```python
from build123d import *

# Parameters (mm, degrees)
CROQUIS1_R              = 1.500000078
CROQUIS1_R_2            = 0.899999978
CROQUIS1_R_3            = 0.899999104
CROQUIS1_R_4            = 1.499997939
CROQUIS1_R_5            = 1.500000378
SALIENTE_EXTRUIR1_DEPTH = 4
CROQUIS2_R              = 1.500000078
CROQUIS2_R_2            = 0.899999978
CROQUIS2_R_3            = 0.899999104
SALIENTE_EXTRUIR2_DEPTH = 4
CROQUIS3_W              = 35.500002289
CROQUIS3_H              = 4.004000187
SALIENTE_EXTRUIR3_DEPTH = 4
CROQUIS4_W              = 38.100002289
CROQUIS4_H              = 4.004000187
SALIENTE_EXTRUIR4_DEPTH = 8
CROQUIS5_R              = 3
CORTAR_EXTRUIR1_DEPTH   = 8


with BuildPart() as part:
    # Croquis1 → Saliente-Extruir1 (new body)
    with BuildSketch(Plane(origin=(0, 0, 0), x_dir=(1, 0, 0), z_dir=(0, 1, 0))):
        with BuildLine():
            Line((-19.24526482, -19.128405422), (20.25473518, -19.128405422))
            ThreePointArc((20.25473518, -19.128405422), (23.250093999, -17.982284574), (24.715306469, -15.12940535))
            Line((24.715306469, -15.12940535), (24.75473518, 3.871594578))
            ThreePointArc((24.75473518, 3.871594578), (24.41495197, 5.657410091), (23.436719128, 7.189614445))
            Line((23.436719128, 7.189614445), (9.132638286, 18.858517697))
            ThreePointArc((9.132638286, 18.858517697), (7.79788024, 19.61076911), (6.288102337, 19.871598393))
            Line((6.288102337, 19.871598393), (-5.278630069, 19.871598393))
            ThreePointArc((-5.278630069, 19.871598393), (-7.047350485, 19.518737385), (-8.545265011, 18.514180332))
            Line((-8.545265011, 18.514180332), (-22.427247654, 7.189612922))
            ThreePointArc((-22.427247654, 7.189612922), (-23.487263037, 5.764725879), (-23.74526482, 4.007634312))
            Line((-23.74526482, 4.007634312), (-23.68986282, -15.332360357))
            ThreePointArc((-23.68986282, -15.332360357), (-22.167781266, -18.050232235), (-19.24526482, -19.128405422))
        make_face()
        with Locations((-10.945264306, -0.628405976)):
            Circle(CROQUIS1_R, mode=Mode.SUBTRACT)
        with Locations((-6.745264379, -0.628405738)):
            Circle(CROQUIS1_R_2, mode=Mode.SUBTRACT)
        with Locations((21.754736572, -0.628405422)):
            Circle(CROQUIS1_R_3, mode=Mode.SUBTRACT)
        with Locations((6.25473312, 16.341597706)):
            Circle(CROQUIS1_R_4, mode=Mode.SUBTRACT)
        with Locations((-4.945262866, 16.341595261)):
            Circle(CROQUIS1_R_5, mode=Mode.SUBTRACT)
        Polygon((-3.845263294, 5.821595341), (-3.74526482, -15.124405235), (5.25473518, -15.124405235), (5.25473518, -7.078405231), (18.854737469, -7.078405231), (18.854737469, 5.821595341), align=None, mode=Mode.SUBTRACT)
    extrude(amount=SALIENTE_EXTRUIR1_DEPTH)

    # Croquis2 → Saliente-Extruir2 (add)
    with BuildSketch(Plane(origin=(0, 4, 0), x_dir=(1, 0, 0), z_dir=(0, 1, 0))):
        with BuildLine():
            Line((-3.74526482, -15.124405235), (-3.835972877, 3.875594765))
            Line((-3.835972877, 3.875594765), (-14.735972877, 3.875594765))
            Line((-14.735972877, 3.875594765), (-14.735972877, -15.124405235))
            Line((-14.735972877, -15.124405235), (-19.24526482, -15.124405235))
            Line((-19.24526482, -15.124405235), (-19.24526482, -19.128405422))
            Line((-19.24526482, -19.128405422), (20.25473518, -19.128405422))
            ThreePointArc((20.25473518, -19.128405422), (23.250093999, -17.982284574), (24.715306469, -15.12940535))
            Line((24.715306469, -15.12940535), (24.75473518, 3.871594578))
            Line((24.75473518, 3.871594578), (18.854737469, 3.871594578))
            Line((18.854737469, 3.871594578), (18.854737469, -7.078405231))
            Line((18.854737469, -7.078405231), (18.854737469, -15.124405235))
            Line((18.854737469, -15.124405235), (5.25473518, -15.124405235))
            Line((5.25473518, -15.124405235), (-3.74526482, -15.124405235))
        make_face()
        with Locations((-10.945264306, -0.628405976)):
            Circle(CROQUIS2_R, mode=Mode.SUBTRACT)
        with Locations((-6.745264379, -0.628405738)):
            Circle(CROQUIS2_R_2, mode=Mode.SUBTRACT)
        with Locations((21.754736572, -0.628405422)):
            Circle(CROQUIS2_R_3, mode=Mode.SUBTRACT)
    extrude(amount=SALIENTE_EXTRUIR2_DEPTH)

    # Croquis3 → Saliente-Extruir3 (add)
    with BuildSketch(Plane(origin=(0, 8, 0), x_dir=(1, 0, 0), z_dir=(0, 1, 0))):
        with Locations((-1.495263676, -17.126405328)):
            Rectangle(CROQUIS3_W, CROQUIS3_H)
    extrude(amount=SALIENTE_EXTRUIR3_DEPTH)

    # Croquis4 → Saliente-Extruir4 (add)
    with BuildSketch(Plane.XZ):
        with Locations((-0.195263676, 17.126405328)):
            Rectangle(CROQUIS4_W, CROQUIS4_H)
    extrude(amount=SALIENTE_EXTRUIR4_DEPTH)

    # Croquis5 → Cortar-Extruir1 (cut)
    with BuildSketch(Plane.XY.offset(19.128405422)):
        with Locations((-0.195262531, 2)):
            Circle(CROQUIS5_R)
        Polygon((16.254737469, 8), (12.254737469, 12), (16.254737469, 12), align=None)
        Polygon((-19.24526482, 4), (-11.24526482, 12), (-19.24526482, 12), align=None)
        Polygon((-19.24526482, 0), (-11.24526482, -8), (-19.24526482, -8), align=None)
        Polygon((18.854737469, -8), (10.854737469, -8), (18.854737469, 0), align=None)
    extrude(amount=-CORTAR_EXTRUIR1_DEPTH, mode=Mode.SUBTRACT)


solid = part.part
```
The listing builds one solid part. Answer for the finished solid, in the listing's coordinates (mm). A direction names the side the tool comes from. Give positions to 0.01 mm unless a question says otherwise; leave off trailing zeros. Order: outer loops, then holes, each group sorted by start corner. A loop starts at its lowest first (then second) coordinate and runs counter-clockwise, first axis right, second up. Notation, with made-up numbers: M -27.5,19.5 L 24.5,19.5 A8 ccw 24.5,27.5 Z; hole C 87,79 d8. An arc over 180 degrees is marked long. Put each result on its own line as item: value. Start each with the question number.
Item 1: The part is cut by section B-B, the plane z = -17. Determine the outline of the cut face in (x, y), and give its area (3 significant figures).
Item 2: Which of the six approach directions +Z, -Z, +X, -X, +Y, -Y give full straight-line access (tool end or side, diameter ignored) to faces 4 (the face through (-2.406, 4.028, 17.154)), 5 (the face through (21, 8, 7)), 6 (the face through (-14.736, 6, 5))?
Item 3: The part is cut by section A-A, the plane z = 13.5. Determine the outline of the cut face in (x, y), and give its area (3 significant figures).
Item 4: Find the intervals of material crossed by line 1 along X through (y, z) = (6.25, 14); line 2 along Z through (x, y) = (1.5, 9.25); line 3 along Y through (x, z) = (-14, -5.5), in increasing order.
Item 5: The part is cut by section C-C, the plane y = 2. Determine the outline of the cut face in (x, z), and give its area (3 significant figures).
Item 6: For a pull along Z with two mould halves and no side action, classify faces 1 (the face through (14.799, -4.056, 17.154)), 2 (the face through (16.385, 1.972, -12.942)), 3 (the face through (7.685, 1.972, -16.792)) as +Z half, -Z half, draft (parallel to the pull), parting line (faces both ways), or undercut.
Item 7: Flat-ended cylindrical pins translate along their axes: P1, Ø1.2, axis at x = -8.5, y = 5.5, coming from the -Z side; P2, Ø2.5, axis at y = 4.5, z = 6, coming from the -X side; P3, Ø5, axis at x = 6.25, z = -16.34, coming from the -Y side; P4, Ø1.1, axis at x = -6.75, z = 0.63, coming from the -Y side. Find the tip coordinate at first contact, or state that the pin passes through.
Item 8: The part is cut by section D-D, the plane z = 9. Determine the outline of the cut face in (x, y), and give its area (3 significant figures).
Answer key:
1. outline: M -10.4,0 L -6.29,0 L -6.29,4 L -10.4,4 Z; M -3.6,0 L 4.91,0 L 4.91,4 L -3.6,4 Z; M 7.6,0 L 11.41,0 L 11.41,4 L 7.6,4 Z
1. area: 65.7 mm²
2. face 4: +Z
2. face 5: +Z, -Z, +X, +Y
2. face 6: -Z, -X, +Y
3. outline: M -23.7,0 L -3.75,0 L -3.75,8 L -14.74,8 L -14.74,4 L -23.7,4 Z; M 5.25,0 L 24.72,0 L 24.72,8 L 18.85,8 L 18.85,4 L 5.25,4 Z
3. area: 225 mm²
4. line 1: x = -14.74 to -3.75, 18.85 to 24.72
4. line 2: z = 15.12 to 19.13
4. line 3: y = 0 to 4
5. outline: M -23.75,-4.01 A3.63 ccw -22.43,-7.19 L -8.55,-18.51 A4.61 ccw -5.28,-19.87 L 6.29,-19.87 A4.5 ccw 9.13,-18.86 L 23.44,-7.19 A4.81 ccw 24.75,-3.87 L 24.72,15.13 A4.49 ccw 20.25,19.13 L 2.8,19.13 L 2.8,15.12 L 5.25,15.12 L 5.25,7.08 L 18.85,7.08 L 18.85,-5.82 L -3.85,-5.82 L -3.75,15.12 L -3.2,15.12 L -3.2,19.13 L -19.25,19.13 A4.5 ccw -23.69,15.33 Z; hole C -10.95,0.63 d3; hole C -6.75,0.63 d1.8; hole C -4.95,-16.34 d3; hole C 6.25,-16.34 d3; hole C 21.75,0.63 d1.8
5. area: 1,230 mm²
6. face 1: draft
6. face 2: -Z half
6. face 3: undercut
7. P1: stops at z = -3.88
7. P2: stops at x = -23.72
7. P3: stops at y = 0
7. P4: passes through
8. outline: M -23.71,0 L -3.77,0 L -3.77,8 L -14.74,8 L -14.74,4 L -23.71,4 Z; M 5.25,0 L 24.73,0 L 24.73,8 L 18.85,8 L 18.85,4 L 5.25,4 Z
8. area: 225 mm²
